Build history of the part. All positions in model axes, mm. Round coordinates to 2 decimals unless told otherwise and drop trailing zeros. Loops run counter-clockwise (first coordinate to the right, second up) from the corner with the lowest first, then second, coordinate; pieces in that order, holes last. Notation, with made-up numbers: (60.25, -32) - (116.25, -32) arc R28 ccw to (116.25, 5) - close; hole circle Ø9 at (29.25, 39). An arc over 180 degrees is marked (long way). Use one line per item in the form item = value. Start each with the question number.
Q1. Pin check, flat tips, straight feed: pin 1 (3 mm diameter, centred on x = -12.793, z = 154.25, fed in from +Y); pin 2 (5 mm diameter, centred on x = -13.5, z = 12.5, fed in from -Y). Stop position of each tip, or through.
Q2. Drill centre lines: line 1 (Z direction, x = -36.5, y = 0.5); line 2 (X direction, y = 3.5, z = -0.5); line 3 (Z direction, x = 14, y = 5.5). Where is each one in solid material? Low to high.
Q3. Saw through at A-A (z = -88.9). Give the cut face in (x, y), then the cut area to 3 significant figures.
Q4. Saw through at B-B (y = 4.5). Count the separate pieces of the cut face and the enclosed holes in it, then the cut area to 3 significant figures.
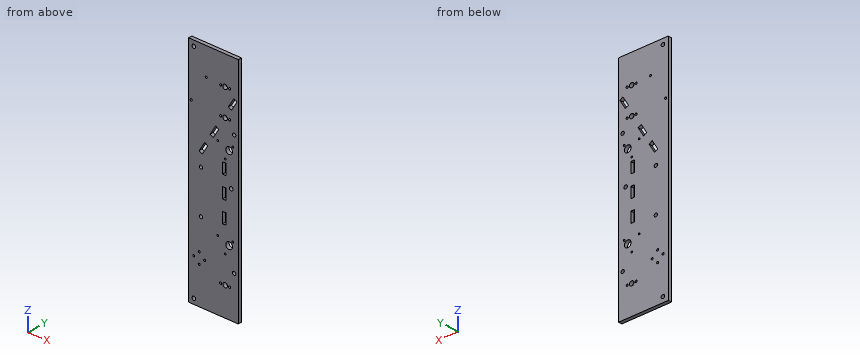
Autodesk Inventor part; units mm, degrees
ref_plane "YZ Plane" through (0, 0, 0) normal (1, 0, 0) x (0, 1, 0)
ref_plane "XZ Plane" through (0, 0, 0) normal (0, 1, 0) x (-1, 0, 0)
ref_plane "XY Plane" through (0, 0, 0) normal (0, 0, 1) x (1, 0, 0)
sketch "Sketch1" plane through (0, 0, 0) normal (0, 1, 0) x (-1, 0, 0)
  line L0 (44.45, 203.2) -> (-44.45, 203.2)
  line L1 (-44.45, 203.2) -> (-44.45, -203.2)
  line L2 (-44.45, -203.2) -> (44.45, -203.2)
  line L3 (44.45, -203.2) -> (44.45, 203.2)
  line L4 (44.45, 203.2) -> (-44.45, -203.2) construction
  line L5 (-44.45, 203.2) -> (-20.955, 203.2)
  line L6 (-20.955, 203.2) -> (-20.955, 88.9) construction
  line L7 (-44.45, 88.9) -> (-44.45, 203.2)
  line L8 (44.45, 203.2) -> (44.45, 111.6492)
  line L9 (44.45, 203.2) -> (44.45, 38.1)
  line L10 (44.45, 38.1) -> (22.225, 38.1) construction
  line L11 (0, 203.2) -> (-66.675, 203.2)
  line L12 (-66.675, 203.2) -> (-66.675, 88.9) construction
  line L13 (-66.675, 203.2) -> (-66.675, 209.55) construction
  line L14 (-20.955, 114.3) -> (-20.955, 152.4) construction
  circle A0 centre (-20.955, 152.4) radius 8.001 construction
  circle A1 centre (-20.955, 152.4) radius 4.0005
  circle A2 centre (-20.955, 160.401) radius 1.85
  line L15 (17.145, 152.4) -> (-20.955, 152.4) construction
  circle A3 centre (-28.956, 152.4) radius 1.85
  line L16 (-20.955, 190.5) -> (-20.955, 152.4) construction
  circle A4 centre (-20.955, 144.399) radius 1.85
  line L17 (-59.055, 152.4) -> (-20.955, 152.4) construction
  circle A5 centre (-12.954, 152.4) radius 1.85
  line L18 (44.45, 0) -> (-44.45, 0) construction
  circle A6 centre (22.225, -63.5) radius 2.9766
  line L19 (32.5679, 18.912) -> (22.7595, 35.2429) construction
  line L20 (22.7595, 35.2429) -> (17.8553, 43.4083) construction
  line L21 (15.6729, 53.2085) -> (25.4813, 36.8776)
  line L22 (25.4813, 36.8776) -> (20.0377, 33.6081)
  line L23 (20.0377, 33.6081) -> (10.2292, 49.939)
  line L24 (10.2292, 49.939) -> (15.6729, 53.2085)
  line L25 (15.6729, 53.2085) -> (20.0377, 33.6081) construction
  line L26 (25.4813, 36.8776) -> (10.2292, 49.939) construction
  circle A7 centre (-20.955, -104.394) radius 1.5
  circle A8 centre (-34.3732, -81.153) radius 1.5
  circle A9 centre (-7.5368, -81.153) radius 1.5
  circle A10 centre (-28.067, -88.9) radius 5.9944
  circle A11 centre (-20.955, -152.4) radius 4.0005
  circle A12 centre (-28.956, -152.4) radius 1.85
  circle A13 centre (-12.954, -152.4) radius 1.85
  circle A14 centre (-37.0613, -128.2) radius 2.9766
  line L27 (-28.067, 88.9) -> (-44.45, 88.9) construction
  line L28 (-44.45, 88.9) -> (-44.45, 12.7)
  line L29 (44.45, 203.2) -> (34.925, 203.2)
  line L30 (34.925, 203.2) -> (34.925, 193.675) construction
  line L31 (34.925, 193.675) -> (44.45, 193.675) construction
  line L32 (44.45, 193.675) -> (44.45, 203.2)
  circle A15 centre (34.925, 193.675) radius 3.175
  line L33 (-44.45, 0) -> (-31.75, 0)
  circle A16 centre (-31.75, 0) radius 3.175
  circle A17 centre (34.925, -193.675) radius 3.175
  line L34 (-44.45, 0) -> (-19.455, 0) construction
  line L35 (-16.28, -76.0639) -> (-22.63, -76.0639) construction
  line L36 (-22.63, -76.0639) -> (-22.63, 51.9267) construction
  line L37 (-22.63, 51.9267) -> (-16.28, 51.9267) construction
  line L38 (-16.28, 51.9267) -> (-16.28, -76.0639) construction
  line L39 (-16.28, -2.5436) -> (-22.63, -2.5436)
  line L40 (-22.63, -2.5436) -> (-22.63, -21.5936)
  line L41 (-22.63, -21.5936) -> (-16.28, -21.5936)
  line L42 (-16.28, -21.5936) -> (-16.28, -2.5436)
  line L43 (-16.28, -40.6436) -> (-22.63, -40.6436)
  line L44 (-16.28, -59.6936) -> (-16.28, -40.6436)
  line L45 (-22.63, -40.6436) -> (-22.63, -59.6936)
  line L46 (-22.63, -59.6936) -> (-16.28, -59.6936)
  line L47 (-16.28, 35.5564) -> (-22.63, 35.5564)
  line L48 (-16.28, 16.5064) -> (-16.28, 35.5564)
  line L49 (-22.63, 35.5564) -> (-22.63, 16.5064)
  line L50 (-22.63, 16.5064) -> (-16.28, 16.5064)
  line L51 (-16.28, -2.5436) -> (-22.63, -2.5436)
  line L52 (-16.28, -21.5936) -> (-16.28, -2.5436)
  line L53 (-22.63, -2.5436) -> (-22.63, -21.5936)
  line L54 (-22.63, -21.5936) -> (-16.28, -21.5936)
  line L55 (44.45, -203.2) -> (25.4, -203.2)
  line L56 (25.4, -203.2) -> (25.4, -128.2) construction
  line L57 (25.4, -128.2) -> (44.45, -128.2) construction
  line L58 (44.45, -128.2) -> (44.45, -203.2)
  circle A18 centre (25.4, -128.2) radius 6.35 construction
  circle A19 centre (25.4, -128.2) radius 9.779 construction
  circle A20 centre (15.621, -128.2) radius 1.778
  circle A21 centre (25.4, -128.2) radius 6.35 construction
  circle A22 centre (25.4, -128.2) radius 9.779 construction
  line L59 (100.4, -128.2) -> (25.4, -128.2) construction
  line L60 (25.4, -128.2) -> (25.4, -109.15) construction
  circle A23 centre (25.4, -137.979) radius 1.778
  circle A24 centre (25.4, -128.2) radius 6.35 construction
  circle A25 centre (25.4, -128.2) radius 9.779 construction
  line L61 (25.4, -53.2) -> (25.4, -128.2) construction
  line L62 (25.4, -128.2) -> (6.35, -128.2) construction
  circle A26 centre (35.179, -128.2) radius 1.778
  circle A27 centre (25.4, -128.2) radius 6.35 construction
  circle A28 centre (25.4, -128.2) radius 9.779 construction
  line L63 (-49.6, -128.2) -> (25.4, -128.2) construction
  line L64 (25.4, -128.2) -> (25.4, -147.25) construction
  circle A29 centre (25.4, -118.421) radius 1.778
  line L65 (22.225, 12.7) -> (22.225, 38.1) construction
  line L66 (-66.675, 209.55) -> (-66.675, 184.15) construction
  circle A30 centre (22.225, 12.7) radius 2.9718
  circle A31 centre (22.225, 12.7) radius 12.065 construction
  line L67 (-20.955, 152.4) -> (-20.955, 104.775) construction
  circle A32 centre (-20.955, 104.775) radius 8.001 construction
  circle A33 centre (-20.955, 112.776) radius 1.8542
  circle A34 centre (-20.955, 104.775) radius 8.001 construction
  circle A35 centre (-28.956, 104.775) radius 1.8542
  circle A36 centre (-20.955, 104.775) radius 8.001 construction
  circle A37 centre (-20.955, 96.774) radius 1.8542
  circle A38 centre (-20.955, 104.775) radius 8.001 construction
  circle A39 centre (-12.954, 104.775) radius 1.8542
  circle A40 centre (-20.955, 152.4) radius 31.75 construction
  circle A41 centre (-20.955, 104.775) radius 15.875 construction
  line L68 (-20.955, 104.775) -> (-20.955, 57.15) construction
  arc A42 (-34.3732, -81.153) -> (-7.5368, -81.153) centre (-20.955, -88.9) ccw construction
  circle A43 centre (-28.067, 57.15) radius 5.9944
  circle A44 centre (-20.955, 41.656) radius 1.5
  circle A45 centre (-7.5368, 64.897) radius 1.5
  circle A46 centre (-34.3732, 64.897) radius 1.5
  arc A47 (-34.3732, 64.897) -> (-7.5368, 64.897) centre (-20.955, 57.15) ccw construction
  circle A48 centre (-20.955, 57.15) radius 31.75 construction
  circle A49 centre (-20.955, -88.9) radius 31.75 construction
  circle A50 centre (-20.955, -152.4) radius 31.75 construction
  line L69 (-3.944, 85.8702) -> (-36.606, 140.3261) construction
  line L70 (-36.606, 140.3261) -> (-26.8074, 123.9893)
  line L71 (-26.8074, 123.9893) -> (-32.253, 120.7231)
  line L72 (-32.253, 120.7231) -> (-42.0516, 137.0599)
  line L73 (-42.0516, 137.0599) -> (-36.606, 140.3261)
  line L74 (-3.944, 85.8702) -> (5.8645, 69.5394)
  line L75 (-9.3876, 82.6008) -> (-3.944, 85.8702)
  line L76 (0.4208, 66.2699) -> (-9.3876, 82.6008)
  line L77 (5.8645, 69.5394) -> (0.4208, 66.2699)
  line L78 (-23.5608, 118.532) -> (-13.7524, 102.2011)
  line L79 (-29.0044, 115.2625) -> (-23.5608, 118.532)
  line L80 (-19.196, 98.9316) -> (-29.0044, 115.2625)
  line L81 (-13.7524, 102.2011) -> (-19.196, 98.9316)
  line L82 (-34.647, 137.0599) -> (7.8217, 162.5369) construction
  line L83 (7.8217, 162.5369) -> (43.4289, 103.1818) construction
  line L84 (43.4289, 103.1818) -> (0.9602, 77.7048) construction
  circle A51 centre (39.6875, 109.4185) radius 1.85
  circle A52 centre (12.793, 154.25) radius 1.85
  circle A53 centre (-20.955, 104.775) radius 4.0005
  circle A54 centre (-37.0613, -128.2) radius 13.335 construction
  line L85 (-37.0613, -128.2) -> (-37.0613, -128.2) construction
  circle A55 centre (-37.0613, 84.5115) radius 2.9766
  circle A56 centre (-37.0613, 84.5115) radius 13.335 construction
  point P0 (0, 0)
  point P1 (-19.455, -12.0686)
  point P2 (-34.2357, -82.6467)
  point P3 (-35.8454, -80.8658)
  dimension "d19" = 16.002
  dimension "d74" = 19.558
  dimension "d112" = 16.002
  dimension "d0" = 88.9
  dimension "d1" = 406.4
  dimension "d5" = 165.1
  dimension "d10" = 6.35
  dimension "d18" = 38.1
  dimension "d20" = 8.001
  dimension "d21" = 3.7
  dimension "d24" = 360
  dimension "d33" = 9.525
  dimension "d34" = 6.35
  dimension "d50" = 9.525
  dimension "d51" = 9.525
  dimension "d52" = 6.35
  dimension "d53" = 12.7
  dimension "d54" = 6.35
  dimension "d57" = 6.35
  dimension "d58" = 127.9906
  dimension "d59" = 6.35
  dimension "d60" = 19.05
  dimension "d63" = 38.1
  dimension "d66" = 38.1
  dimension "d71" = 75
  dimension "d72" = 19.05
  dimension "d73" = 12.7
  dimension "d75" = 3.556
  dimension "d78" = 360
  dimension "d84" = 25.4
  dimension "d85" = 5.9436
  dimension "d86" = 24.13
  dimension "d87" = 19.05
  dimension "d110" = 47.625
  dimension "d113" = 3.7084
  dimension "d116" = 360
  dimension "d118" = 63.5
  dimension "d119" = 31.75
  dimension "d120" = 47.625
  dimension "d135" = 63.5
  dimension "d136" = 63.5
  dimension "d137" = 63.5
  dimension "d138" = 63.5
  dimension "d139" = 19.05
  dimension "d140" = 6.35
  dimension "d143" = 38.1
  dimension "d150" = 3.7
  dimension "d151" = 3.7
  dimension "d154" = 8.001
  dimension "d157" = 26.67
  dimension "d178" = 26.67
extrude "Extrusion13" add sketch "Sketch1" along normal blind 6.35 contours L3 L2 L1 L0 | A2 | A4 | A33 L78 | L78 A33 | A33 L78 L81 L80 A53 L79 | A37
properties part number "ChassisOutide10"
Report:
q1.pin_1 = through
q1.pin_2 = 0
q2.line_1 = -203.2 to -196.43, -190.92 to -129.39, -127.01 to 190.92, 196.43 to 203.2
q2.line_2 = -44.45 to 28.61, 34.89 to 44.45
q2.line_3 = -203.2 to -153.93, -150.87 to 103.24, 106.31 to 150.87, 153.93 to 203.2
q3.outline = (-44.45, 0) - (22.07, 0) - (22.07, 6.35) - (-44.45, 6.35) - close; (34.06, 0) - (44.45, 0) - (44.45, 6.35) - (34.06, 6.35) - close
q3.area = 488 mm²
q4.separate_pieces = 1
q4.enclosed_holes = 36
q4.area = 34,700 mm²
